Verification items for this drawing (mm, ordinates from the low corner). A direction names the side the tool comes from. Round coordinates to 2 decimals unless told otherwise and drop trailing zeros. Order: outer loops, then holes, each group sorted by start corner. A loop starts at its lowest first (then second) coordinate and runs counter-clockwise, first axis right, second up. Notation, with made-up numbers: (42, -29.75) - (71, -29.75) arc R18 ccw to (71, -12.75) - close; hole circle Ø8 at (-20, -23). An arc over 180 degrees is marked (long way). One line per question, with ' | ' between items. Start each with the question number.
Q1. Material ranges on line 1 along Y through (x, z) = (3, 2); line 2 along X through (y, z) = (18.5, 2); line 3 along X through (y, z) = (15.25, 15), recorded low to high.
Q2. Sectioned sample at B-B, the plane z = 2.5. Enter the section's corners in (x, y).
Q3. Tool access check on the marked faces 5, 6 and 7. Record the directions out of +Z, -Z, +X, -X, +Y, -Y that give a thin tool (end or side, any length) a straight path to the whole face; none if there is none.
Q4. Mould release check, pull along X, two halves, no side actions. Record for the marked faces 1, 2, 3 and 4: +X half, -X half, draft (parallel to the pull), parting line (faces both ways), or undercut.
Q5. Gauge pin test, flat ends, axial feed: P1, Ø6, axis at y = 5.5, z = 13.5, coming from the -X side; P2, Ø10, axis at x = 16, y = 3, coming from the +Z side. Record the tip position at first contact, or that the pin passes through.
Q6. Sectioned sample at C-C, the plane y = 4.5. Enter the section's corners in (x, z).
Q7. Sectioned sample at D-D, the plane z = 28. Enter the section's corners in (x, y), then the cut area to 3 significant figures.
Q8. Sectioned sample at A-A, the plane x = 2.5. Enter the section's corners in (y, z).
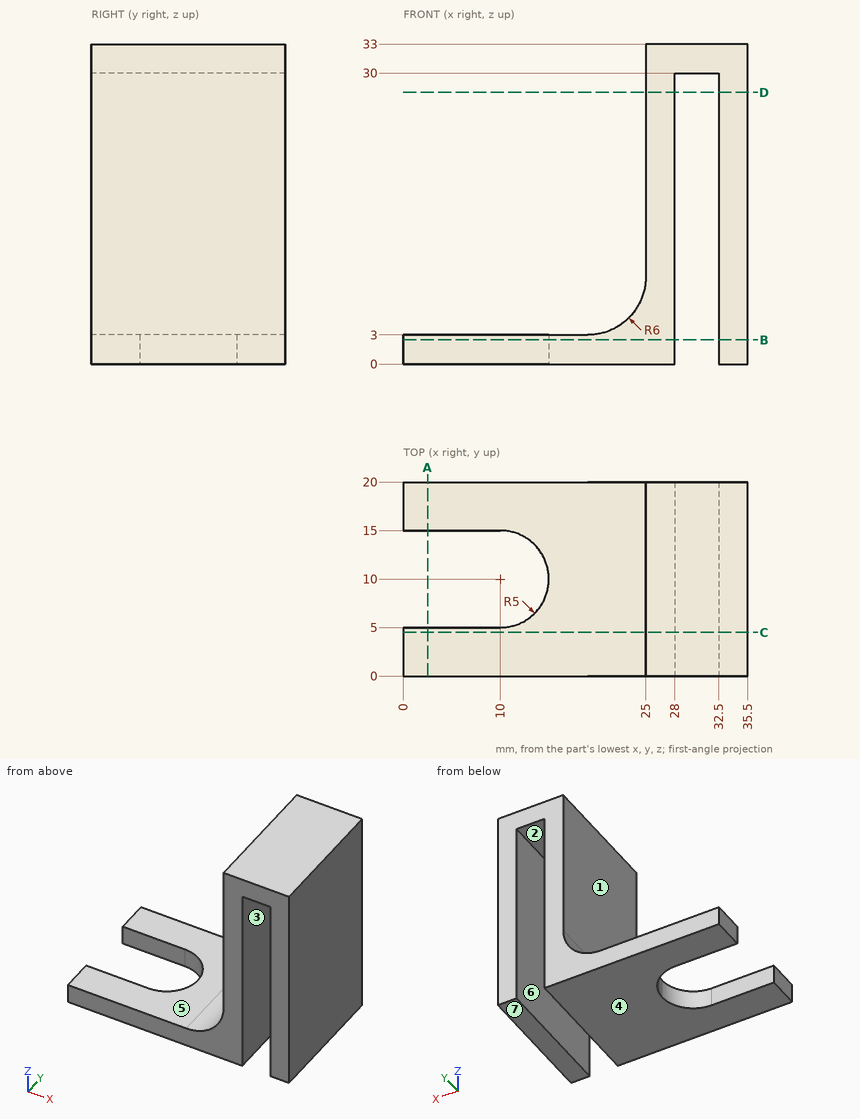
Determined:
1) line 1: y = 0 to 5, 15 to 20 | line 2: x = 0 to 28, 32.5 to 35.5 | line 3: x = 25 to 28, 32.5 to 35.5
2) outline: (0, 0) - (28, 0) - (28, 20) - (0, 20) - (0, 15) - (10, 15) arc R5 cw to (10, 5) - (0, 5) - close; (32.5, 0) - (35.5, 0) - (35.5, 20) - (32.5, 20) - close
3) face 5: +Z, -X, +Y, -Y | face 6: -Z, +Y, -Y | face 7: -Z, +X, -X, +Y, -Y
4) face 1: -X half | face 2: undercut | face 3: undercut | face 4: draft
5) P1: stops at x = 25 | P2: stops at z = 3.34
6) outline: (0, 0) - (28, 0) - (28, 30) - (32.5, 30) - (32.5, 0) - (35.5, 0) - (35.5, 33) - (25, 33) - (25, 9) arc R6 cw to (19, 3) - (0, 3) - close
7) outline: (25, 0) - (28, 0) - (28, 20) - (25, 20) - close; (32.5, 0) - (35.5, 0) - (35.5, 20) - (32.5, 20) - close | area: 120 mm2
8) outline: (0, 0) - (5, 0) - (5, 3) - (0, 3) - close; (15, 0) - (20, 0) - (20, 3) - (15, 3) - close
